The listing builds one solid part. Answer for the finished solid, in the listing's coordinates (mm). A direction names the side the tool comes from. Coordinates: 2 decimals unless noted, no trailing zeros. Use a Markdown table: item, result. Add a question column.
Item 1: Flat-ended cylindrical pins translate along their axes: P1, Ø6.5, axis at x = -5, y = 0, coming from the -Z side; P2, Ø12, axis at y = -5, z = 10, coming from the -X side; P3, Ø14, axis at x = -5, y = -7, coming from the -Z side; P4, Ø1.9, axis at x = -3, z = 17, coming from the -Y side. Find the tip coordinate at first contact, or state that the pin passes through.
Item 2: Find the intervals of material crossed by line 1 along X through (y, z) = (4.75, 19.5); line 2 along X through (y, z) = (-0.5, 31.5); line 3 along Y through (x, z) = (12, 5.5), in increasing order.
Item 3: For faces 1 (the cylindrical face through (-0.67, 1.29, 44.77)), 2 (the cylindrical face through (0, 13, 27)), 3 (the flat face through (-5, 12.5, 16)), determine the directions among +Z, -Z, +X, -X, +Y, -Y from which every point of the face is accessible in a straight line to the end or side of a thin tool.
Item 4: The mould has two halves that part along Z. Classify faces 4 (the cylindrical face through (0, 7.4, 40.3)), 5 (the flat face through (0, 14, 28)): released by +Z, released by -Z, zero draft, split by the parting line, or undercut.
Item 5: The part is cut by section A-A, the plane x = -5. State how many separate pieces and enclosed holes the cut face has, then the cut area to 3 significant figures.
from build123d import *

# Parameters (mm, degrees)
SKETCH1_W           = 33
SKETCH1_H           = 28
BOSS_EXTRUDE1_DEPTH = 46
CUT_EXTRUDE1_DEPTH  = 59.318093247
CUT_EXTRUDE2_START  = -3
CUT_EXTRUDE2_DEPTH  = 27
FILLET1_R           = 12.5
FILLET2_R           = 16.5
FILLET3_R           = 6
SKETCH6_W           = 13
SKETCH6_H           = 23
CUT_EXTRUDE3_DEPTH  = 9
SKETCH8_R           = 6.5
CUT_EXTRUDE4_DEPTH  = 9
SKETCH9_R           = 1
CUT_EXTRUDE5_DEPTH  = 8
SKETCH10_R          = 1.3
SKETCH10_R_2        = 2.5
CUT_EXTRUDE6_DEPTH  = 2.5


with BuildPart() as part:
    # Sketch1 → Boss-Extrude1 (new body)
    with BuildSketch(Plane.XY):
        Rectangle(SKETCH1_W, SKETCH1_H)
    extrude(amount=BOSS_EXTRUDE1_DEPTH)

    # Sketch3 → Cut-Extrude1 (cut, through all)
    with BuildSketch(Plane.ZY.offset(16.5)):
        with BuildLine():
            Line((0, 2), (0, -14))
            Line((0, -14), (41, -14))
            add(Edge.make_bspline(
                [(41, -14), (21.241610725, -3.748388801), (0, 2)],
                knots=[0, 0, 0, 1, 1, 1], degree=2))
        make_face()
    extrude(amount=-CUT_EXTRUDE1_DEPTH, mode=Mode.SUBTRACT)

    # Sketch4 → Cut-Extrude2 (cut)
    with BuildSketch(Plane.ZY.offset(16.5).offset(CUT_EXTRUDE2_START)):
        with BuildLine():
            Line((41, -14), (43.5, -14))
            Line((43.5, -14), (43.5, 3.5))
            Line((43.5, 3.5), (5.5, 3.5))
            Line((5.5, 3.5), (5.5, 0.428638096))
            add(Edge.make_bspline(
                [(41, -14), (23.811256263, -5.081645607), (5.5, 0.428638096)],
                knots=[0, 0, 0, 1, 1, 1], degree=2))
        make_face()
    extrude(amount=-CUT_EXTRUDE2_DEPTH, mode=Mode.SUBTRACT)

    # Fillet1
    fillet1_edges = [part.edges().sort_by_distance(p)[0] for p in [
        (-13.5, 1.964319048, 5.5),
        (13.5, 1.964319048, 5.5),
    ]]
    fillet(fillet1_edges, radius=FILLET1_R)

    # Fillet2
    fillet2_edges = [part.edges().sort_by_distance(p)[0] for p in [
        (-16.5, 8, 0),
        (16.5, 8, 0),
    ]]
    fillet(fillet2_edges, radius=FILLET2_R - 0.0001)  # a hair under: the kernel refuses the full size

    # Fillet3
    fillet3_edges = [part.edges().sort_by_distance(p)[0] for p in [
        (16.5, -14, 43.5),
        (-16.5, -14, 43.5),
    ]]
    fillet(fillet3_edges, radius=FILLET3_R)

    # Sketch6 → Cut-Extrude3 (cut)
    with BuildSketch(Plane.XZ.offset(-3.5)):
        with Locations((0, 25.5)):
            Rectangle(SKETCH6_W, SKETCH6_H)
    extrude(amount=-CUT_EXTRUDE3_DEPTH, mode=Mode.SUBTRACT)

    # Sketch8 → Cut-Extrude4 (cut)
    with BuildSketch(Plane.XZ.offset(-12.5)):
        with Locations(Location((0, 20.5, 0), (0, 0, 270))):
            Circle(SKETCH8_R)
    extrude(amount=-CUT_EXTRUDE4_DEPTH, mode=Mode.SUBTRACT)

    # Sketch9 → Cut-Extrude5 (cut)
    with BuildSketch(Plane.XZ.offset(-3.5)):
        with Locations(Location((0, 39.3, 0), (0, 0, 270))):
            Circle(SKETCH9_R)
        with Locations(Location((0, 11.7, 0), (0, 0, 270))):
            Circle(SKETCH9_R)
    extrude(amount=-CUT_EXTRUDE5_DEPTH, mode=Mode.SUBTRACT)

    # Sketch10 → Cut-Extrude6 (cut)
    with BuildSketch(Plane.XY.offset(46)):
        with Locations((-9.5, 0)):
            Circle(SKETCH10_R)
        with Locations((-5, 0)):
            Circle(SKETCH10_R_2)
        with Locations((-0.5, 0)):
            Circle(SKETCH10_R)
    extrude(amount=-CUT_EXTRUDE6_DEPTH, mode=Mode.SUBTRACT)


solid = part.part
Solution:
| question | item | result |
|---|---|---|
| 1 | P1 | stops at z = 0.18 |
| 1 | P2 | stops at x = -16.48 |
| 1 | P3 | stops at z = 43.5 |
| 1 | P4 | passes through |
| 2 | line 1 | x = -16.5 to -6.5, 6.5 to 16.5 |
| 2 | line 2 | x = -16.5 to -13.5, 13.5 to 16.5 |
| 2 | line 3 | y = 0.43 to 14 |
| 3 | face 1 | +Z |
| 3 | face 2 | +Y, -Y |
| 3 | face 3 | -Y |
| 4 | face 4 | undercut |
| 4 | face 5 | zero draft |
| 5 | separate pieces | 3 |
| 5 | enclosed holes | 0 |
| 5 | area | 300 mm2 |
